from build123d import *

# Parameters (mm, degrees)
SKETCH1_R           = 1.5
SKETCH1_R_2         = 0.5
BOSS_EXTRUDE1_DEPTH = 3
SKETCH2_R           = 0.5
CUT_EXTRUDE1_DEPTH  = 3


with BuildPart() as part:
    # Sketch1 → Boss-Extrude1 (new body)
    with BuildSketch(Plane(origin=(0, 0, 0), x_dir=(1, 0, 0), z_dir=(0, 1, 0))):
        with BuildLine():
            Line((-1.75, 12.75), (-2.985348867, 0.296128587))
            ThreePointArc((-2.985348867, 0.296128587), (0, -3), (2.985348867, 0.296128587))
            Line((2.985348867, 0.296128587), (1.75, 12.75))
            ThreePointArc((1.75, 12.75), (0, 14.5), (-1.75, 12.75))
        make_face()
        Circle(SKETCH1_R, mode=Mode.SUBTRACT)
        with Locations((0, 5)):
            Circle(SKETCH1_R_2, mode=Mode.SUBTRACT)
        with Locations((0, 7)):
            Circle(SKETCH1_R_2, mode=Mode.SUBTRACT)
        with Locations((0, 9)):
            Circle(SKETCH1_R_2, mode=Mode.SUBTRACT)
        with Locations((0, 11)):
            Circle(SKETCH1_R_2, mode=Mode.SUBTRACT)
        with Locations((0, 13)):
            Circle(SKETCH1_R_2, mode=Mode.SUBTRACT)
    extrude(amount=BOSS_EXTRUDE1_DEPTH)

    # Sketch2 → Cut-Extrude1 (cut)
    with BuildSketch(Plane.XY.offset(3)):
        with Locations((0, 1.5)):
            Circle(SKETCH2_R)
    extrude(amount=-CUT_EXTRUDE1_DEPTH, mode=Mode.SUBTRACT)


solid = part.part
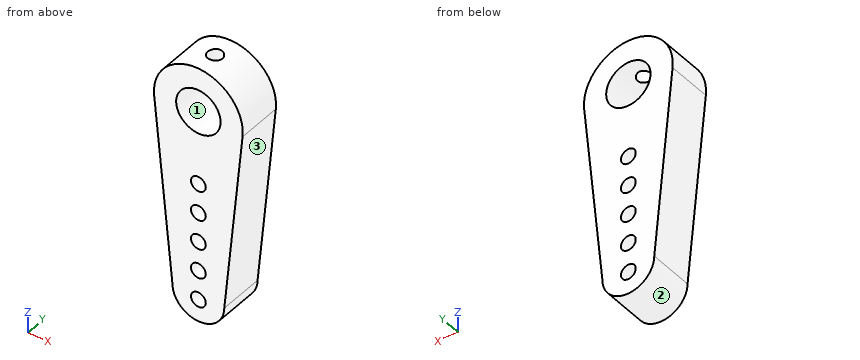
The model under review builds one solid part; all positions refer to its coordinate system, in mm. Face numbers are marked on the shaded views. Give positions to 0.01 mm unless a question says otherwise; leave off trailing zeros. Loops run counter-clockwise (first coordinate to the right, second up) from the corner with the lowest first, then second, coordinate; pieces in that order, holes last. Notation, with made-up numbers: (36, -39) -> (53, -39) arc R9 cw to (53, -23) -> close; hole circle Ø6 at (71, 25). An arc over 180 degrees is marked (long way). Put each result on its own line as item: value. Start each with the question number.
1. Clearance check with flat-ended pins moving along their axes: P1, Ø1.5, axis at x = -2, y = 1.5, coming from the -Z side; P2, Ø1.5, axis at y = 1, z = -1, coming from the +X side; P3, Ø1, axis at y = 1, z = -8, coming from the +X side. State where each tip first meets the part, or that it passes through.
2. We need section C-C on z = 0. State the section outline as (x, y) points, then the cut area to 3 significant figures.
3. Mouldability with a two-part tool opening along X and no side actions: class the marked faces 1, 2 and 3 as released by +X, released by -X, zero draft, split by the parting line, or undercut.
4. We need section D-D on y = 1.5. State the section outline as (x, z) points.
5. We need section B-B on x = 0. State how many separate pieces and enclosed holes the cut face has, then the cut area to 3 significant figures.
6. We need section A-A on y = 0.65. State the section outline as (x, z) points.
7. Wall thickness on probe 1 along Z at (x, y) = (0, 1.9); probe 2 along X at (y, z) = (2.05, 0); probe 3 along Y at (x, z) = (0, 2.65): over which ranges is each line inside the solid? List them lowest first.
Determined:
1. P1: z = -13.97
1. P2: x = 2.99
1. P3: x = 2.27
2. outline: (-3, 0) -> (-1.5, 0) -> (-1.5, 3) -> (-3, 3) -> close; (1.5, 0) -> (3, 0) -> (3, 3) -> (1.5, 3) -> close
2. area: 9.00 mm^2
3. face 1: undercut
3. face 2: split by the parting line
3. face 3: released by +X
4. outline: (-2.99, -0.3) -> (-1.75, -12.75) arc R1.75 ccw to (1.75, -12.75) -> (2.99, -0.3) arc R3 ccw to (0.5, 2.96) -> (0.5, 1.41) arc R1.5 cw (long way) to (-0.5, 1.41) -> (-0.5, 2.96) arc R3 ccw to start; hole circle Ø1 at (0, -13); hole circle Ø1 at (0, -11); hole circle Ø1 at (0, -9); hole circle Ø1 at (0, -7); hole circle Ø1 at (0, -5)
5. separate pieces: 8
5. enclosed holes: 0
5. area: 27.0 mm^2
6. outline: (-2.99, -0.3) -> (-1.75, -12.75) arc R1.75 ccw to (1.75, -12.75) -> (2.99, -0.3) arc R3 ccw (long way) to start; hole circle Ø3 at (0, 0); hole circle Ø1 at (0, -13); hole circle Ø1 at (0, -11); hole circle Ø1 at (0, -9); hole circle Ø1 at (0, -7); hole circle Ø1 at (0, -5)
7. probe 1: -14.5 to -13.5, -12.5 to -11.5, -10.5 to -9.5, -8.5 to -7.5, -6.5 to -5.5, -4.5 to -1.5
7. probe 2: -3 to -1.5, 1.5 to 3
7. probe 3: 0 to 1, 2 to 3
